```python
from build123d import *

# Parameters (mm, degrees)
SKETCH_1_W          = 180
SKETCH_1_H          = 66
EXTRUDE_1_DEPTH     = 3
SKETCH_2_W          = 180
SKETCH_2_H          = 3
EXTRUDE_2_DEPTH     = 50
SKETCH_3_W          = 9
SKETCH_3_H          = 32
EXTRUDE_3_DEPTH     = 30
SKETCH_4_W          = 22
SKETCH_4_H          = 5
SKETCH_4_H_2        = 4.5
EXTRUDE_4_DEPTH     = 12
SKETCH_9_W          = 180
SKETCH_9_H          = 66
EXTRUDE_7_DEPTH     = 30
EXTRUDE_8_DEPTH     = 66
EXTRUDE_9_DEPTH     = 3
EXTRUDE_10_DEPTH    = 3
EXTRUDE_11_DEPTH    = 60
SKETCH_16_R         = 1
CUT_EXTRUDE_1_DEPTH = 15
SKETCH_17_W         = 40.157277222
SKETCH_17_H         = 30
SKETCH_17_W_2       = 44.638770814
CUT_EXTRUDE_2_DEPTH = 67


with BuildPart() as part:
    # 草圖1 → 填料-伸長1 (new body)
    with BuildSketch(Plane.XY):
        with Locations((90, 33)):
            Rectangle(SKETCH_1_W, SKETCH_1_H)
    extrude(amount=EXTRUDE_1_DEPTH)

    # 草圖2 → 填料-伸長2 (add)
    with BuildSketch(Plane.XY.offset(3)):
        with Locations((90, 1.5)):
            Rectangle(SKETCH_2_W, SKETCH_2_H)
        with Locations((90, 64.5)):
            Rectangle(SKETCH_2_W, SKETCH_2_H)
    extrude(amount=EXTRUDE_2_DEPTH)

    # 草圖3 → 填料-伸長3 (add)
    with BuildSketch(Plane.ZY):
        with Locations((4.5, -16)):
            Rectangle(SKETCH_3_W, SKETCH_3_H)
    extrude(amount=-EXTRUDE_3_DEPTH)

    # 草圖4 → 填料-伸長4 (add)
    with BuildSketch(Plane.XY.offset(9)):
        with Locations((19, -2.5)):
            Rectangle(SKETCH_4_W, SKETCH_4_H)
        with Locations((19, -29.75)):
            Rectangle(SKETCH_4_W, SKETCH_4_H_2)
    extrude(amount=EXTRUDE_4_DEPTH)

    # 草圖9 → 填料-伸長7 (add)
    with BuildSketch(Plane(origin=(0, 0, 0), x_dir=(-1, 0, 0), z_dir=(0, 0, -1))):
        with Locations((-90, 33)):
            Rectangle(SKETCH_9_W, SKETCH_9_H)
    extrude(amount=EXTRUDE_7_DEPTH)

    # 草圖10 → 填料-伸長8 (add)
    with BuildSketch(Plane.XZ):
        Polygon((0, 0), (180, 0), (180, 68.514642168), (0, 3), align=None)
    extrude(amount=-EXTRUDE_8_DEPTH)

    # 草圖11 → 填料-伸長9 (add)
    with BuildSketch(Plane.XZ):
        Polygon((180, 68.514642168), (180, 118.514642168), (0, 53), (137.373870973, 53), align=None)
    extrude(amount=-EXTRUDE_9_DEPTH)

    # 草圖12 → 填料-伸長10 (add)
    with BuildSketch(Plane(origin=(0, 66, 0), x_dir=(1, 0, 0), z_dir=(0, 1, 0))):
        Polygon((180, -68.514642168), (180, -118.514642168), (0, -53), (137.373870973, -53), align=None)
    extrude(amount=-EXTRUDE_10_DEPTH)

    # 草圖14 → 填料-伸長11 (add)
    with BuildSketch(Plane.XZ.offset(-63)):
        Polygon((180, 118.514642168), (180, 68.514642168), (177.180922138, 67.488581738), (177.180922138, 117.488581738), align=None)
    extrude(amount=EXTRUDE_11_DEPTH)

    # 草圖16 → 除料-伸長1 (cut)
    with BuildSketch(Plane.ZY.offset(-8)):
        with Locations((15, -2.5)):
            Circle(SKETCH_16_R)
        with Locations((15, -30)):
            Circle(SKETCH_16_R)
    extrude(amount=-CUT_EXTRUDE_1_DEPTH, mode=Mode.SUBTRACT)

    # 草圖17 → 除料-伸長2 (cut, through all)
    with BuildSketch(Plane.XZ):
        with Locations((20.078638611, -15)):
            Rectangle(SKETCH_17_W, SKETCH_17_H)
        with Locations((157.680614593, -15)):
            Rectangle(SKETCH_17_W_2, SKETCH_17_H)
    extrude(amount=-CUT_EXTRUDE_2_DEPTH, mode=Mode.SUBTRACT)


solid = part.part
```
The listing builds one solid part. Answer for the finished solid, in the listing's coordinates (mm). A direction names the side the tool comes from. Give positions to 0.01 mm unless a question says otherwise; leave off trailing zeros. Write each loop counter-clockwise with the first axis right and the second up, starting at its lowest first coordinate (ties: lowest second). Pieces come first, ordered by that corner, then holes. Notation, with made-up numbers: M -37,-7 L 15,-7 A13 cw 15,4 Z; hole C 79.25,30 d1. An arc over 180 degrees is marked long. Write each question's results on one line, items separated by ' | '.
Q1. For a pull along Y with two mould halves and no side action, classify faces 5 (the flat face through (87, 3, 61)), 6 (the flat face through (19, -30, 21)), 7 (the flat face through (91, 66, 43)) as released by +Y, released by -Y, zero draft, split by the parting line, or undercut.
Output values:
face 5: undercut | face 6: zero draft | face 7: released by +Y
Q2. Consider L1, parallel to Y at x = 13.5, z = 15; L2, parallel to Y at x = 73, z = 73.5; L3, parallel to Y at x = 84, z = -18. Determine where each line is inside the solid, lowest interval first. Write a range as from..to.
Output values:
L1: -32..-31, -29..-27.5, -5..-3.5, -1.5..3, 63..66 | L2: 0..3, 63..66 | L3: 0..66
Q3. Flat-ended cylindrical pins translate along their axes: P1, Ø2.5, axis at x = 23.5, y = -2, coming from the +Z side; P2, Ø4, axis at x = 56, z = 3.5, coming from the -Y side; P3, Ø1.6, axis at y = -2.5, z = 15, coming from the -X side. Find the tip coordinate at first contact, or state that the pin passes through.
Output values:
P1: z = 21 | P2: y = 0 | P3: x = 23
Q4. Section D-D, the plane y = -20.5 is taken. Write down the section's boundary in (x, z), then the cut area to 3 significant figures.
Output values:
outline: M 0,0 L 30,0 L 30,9 L 0,9 Z | area: 270 mm2
Q5. Section A-A, the plane y = 35.5 is taken. Write down the section's boundary in (x, z).
Output values:
outline: M 0,0 L 40.16,0 L 40.16,-30 L 135.36,-30 L 135.36,0 L 180,0 L 180,118.51 L 177.18,117.49 L 177.18,67.49 L 0,3 Z
Q6. Section C-C, the plane z = -10 is taken. Write down the section's boundary in (x, y), then the cut area to 3 significant figures.
Output values:
outline: M 40.16,0 L 135.36,0 L 135.36,66 L 40.16,66 Z | area: 6,280 mm2
Q7. A tool of negligible diameter and unlimited length cuts with its end or side. For faces 1 (the flat face through (157, 33, 0)), 2 (the flat face through (19, -27.5, 15)), 3 (the flat face through (8, -28.8, 14.9)), 4 (the flat face through (89.831, 32.58, 35.696)), from which of +Z, -Z, +X, -X, +Y, -Y can it reach the whole face along a straight path? Write none if from no direction.
Output values:
face 1: -Z, +X, +Y, -Y | face 2: +Z, +X, -X | face 3: +Z, -X, -Y | face 4: +Z, -X
Q8. Section B-B, the plane z = 63.5 is taken. Write down the section's boundary in (x, y).
Output values:
outline: M 28.85,0 L 180,0 L 180,66 L 28.85,66 L 28.85,63 L 166.22,63 L 166.22,3 L 28.85,3 Z
